```python
from build123d import *

# Parameters (mm, degrees)
CROQUIS1_R              = 50.744242673
SALIENTE_EXTRUIR1_DEPTH = 12
SALIENTE_EXTRUIR2_DEPTH = 12
CROQUIS3_R              = 6.412213352
SALIENTE_EXTRUIR3_DEPTH = 120


with BuildPart() as part:
    # Croquis1 → Saliente-Extruir1 (new body)
    with BuildSketch(Plane(origin=(0, 0, 0), x_dir=(1, 0, 0), z_dir=(0, 1, 0))):
        with Locations(Location((0, 0, 0), (0, 0, 270))):
            Circle(CROQUIS1_R)
    extrude(amount=SALIENTE_EXTRUIR1_DEPTH)

    # Croquis2 → Saliente-Extruir2 (add)
    with BuildSketch(Plane(origin=(0, 12, 0), x_dir=(1, 0, 0), z_dir=(0, 1, 0))):
        Polygon((11.547005384, 0), (5.773502692, 10), (-5.773502692, 10), (-11.547005384, 0), (-5.773502692, -10), (5.773502692, -10), align=None)
    extrude(amount=SALIENTE_EXTRUIR2_DEPTH)

    # Croquis3 → Saliente-Extruir3 (add)
    with BuildSketch(Plane(origin=(0, 24, 0), x_dir=(1, 0, 0), z_dir=(0, 1, 0))):
        with Locations(Location((0, 0, 0), (0, 0, 270))):
            Circle(CROQUIS3_R)
    extrude(amount=SALIENTE_EXTRUIR3_DEPTH)


solid = part.part
```
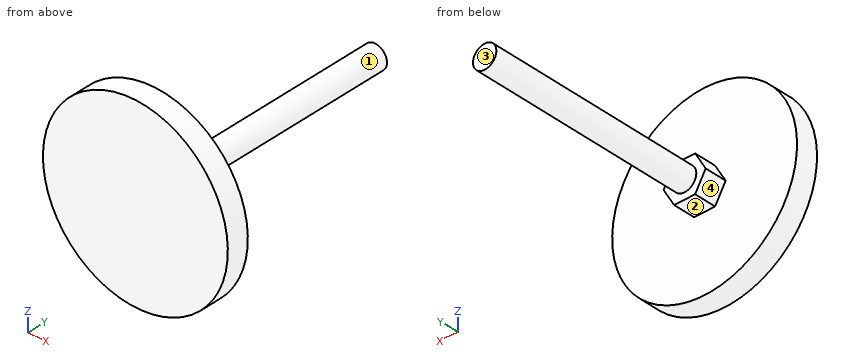
Build history of the part. All positions in model axes, mm. Face numbers are marked on the shaded views. A direction names the side the tool comes from. Coordinates: 2 decimals unless noted, no trailing zeros. Order: outer loops, then holes, each group sorted by start corner. A loop starts at its lowest first (then second) coordinate and runs counter-clockwise, first axis right, second up.
Item 1: Tool access for the marked faces 1, 2, 3 and 4: list every direction of +Z, -Z, +X, -X, +Y, -Y with a clear straight run to the whole face (end or side of a thin tool).
Filled in:
face 1: +Y
face 2: -Z, +X, -X, +Y
face 3: +Z, -Z, +X, -X, +Y
face 4: -Z, -X, +Y
Item 2: Saw through at B-B on y = 92. List the corners of the cut face in (x, z), then the cut area to 3 significant figures.
Filled in:
outline: circle Ø12.82 at (0, 0)
area: 129 mm2
Item 3: Saw through at A-A on x = 0. List the corners of the cut face in (y, z), then the cut area to 3 significant figures.
Filled in:
outline: (0, -50.74) - (12, -50.74) - (12, -10) - (24, -10) - (24, -6.41) - (144, -6.41) - (144, 6.41) - (24, 6.41) - (24, 10) - (12, 10) - (12, 50.74) - (0, 50.74) - close
area: 3,000 mm2
Item 4: Saw through at D-D on x = 23. List the corners of the cut face in (y, z).
Filled in:
outline: (0, -45.23) - (12, -45.23) - (12, 45.23) - (0, 45.23) - close
Item 5: Drop flat-ended pins along their axis: pin 1 Ø1.5 at (x, z) = (-24.5, 19) entering from +Y; pin 2 Ø12.5 at (x, y) = (1, 18.5) entering from +Z; pin 3 Ø3.5 at (x, y) = (0, 17.5) entering from -Z; pin 4 Ø12 at (y, z) = (61.5, -14.5) entering from -X. Give the stop position or say it passes through.
Filled in:
pin 1: stops at y = 12
pin 2: stops at z = 10
pin 3: stops at z = -10
pin 4: passes through
Item 6: Saw through at C-C on z = 19.5. List the corners of the cut face in (x, y).
Filled in:
outline: (-46.85, 0) - (46.85, 0) - (46.85, 12) - (-46.85, 12) - close
Item 7: Drill centre lines: L1, parallel to Y at x = -46, z = -9; L2, parallel to Z at x = -45.5, y = 7; L3, parallel to X at y = 104.5, z = -2. Where is each one in solid material? Low to high.
Filled in:
L1: y = 0 to 12
L2: z = -22.47 to 22.47
L3: x = -6.09 to 6.09
